```python
from build123d import *

# Parameters (mm, degrees)
SKETCH_W        = 55.5
SKETCH_H        = 55.5
SKETCH_R        = 19.25
PAD_DEPTH       = 6
SKETCH001_W     = 58.5
SKETCH001_H     = 8
PAD001_DEPTH    = 5
SKETCH002_W     = 30
SKETCH002_H     = 5
PAD002_DEPTH    = 20
FILLET_R        = 5
POCKET_DEPTH    = 6
FILLET001_R     = 9
FILLET002_R     = 7
CHAMFER_SIZE    = 3
SKETCH004_R     = 19.25
SKETCH004_R_2   = 18.5
PAD003_DEPTH    = 1.5
SKETCH005_W     = 45.5
SKETCH005_H     = 45.5
POCKET001_DEPTH = 3
SKETCH006_R     = 1
POCKET002_DEPTH = 6
FILLET003_R     = 1
FILLET004_R     = 1
SKETCH007_R     = 5
POCKET003_DEPTH = 2.999


with BuildPart() as part:
    # Sketch → Pad (new body)
    with BuildSketch(Plane.XY):
        Rectangle(SKETCH_W, SKETCH_H)
        Circle(SKETCH_R, mode=Mode.SUBTRACT)
    extrude(amount=PAD_DEPTH)

    # Sketch001 → Pad001 (new body)
    with BuildSketch(Plane(origin=(0, 27.75, 0), x_dir=(-1, 0, 0), z_dir=(0, 1, 0))):
        with Locations((0, 3)):
            Rectangle(SKETCH001_W, SKETCH001_H)
    extrude(amount=PAD001_DEPTH)

    # Sketch002 → Pad002 (new body)
    with BuildSketch(Plane(origin=(0, 32.75, 0), x_dir=(-1, 0, 0), z_dir=(0, 1, 0))):
        with Locations((0, 3)):
            Rectangle(SKETCH002_W, SKETCH002_H)
    extrude(amount=PAD002_DEPTH)

    # Fillet
    fillet_edges = [part.edges().sort_by_distance(p)[0] for p in [
        (-27.75, -27.75, 3),
        (27.75, -27.75, 3),
    ]]
    fillet(fillet_edges, radius=FILLET_R)

    # Sketch003 → Pocket (cut)
    with BuildSketch(Plane(origin=(0, 0, 0.5), x_dir=(1, 0, 0), z_dir=(0, 0, -1))):
        with BuildLine():
            ThreePointArc((-5, -36.75), (-11, -42.75), (-5, -48.75))
            Line((-5, -48.75), (5, -48.75))
            ThreePointArc((5, -48.75), (11, -42.75), (5, -36.75))
            Line((-5, -36.75), (5, -36.75))
        make_face()
    extrude(amount=-POCKET_DEPTH, mode=Mode.SUBTRACT)

    # Fillet001
    fillet001_edges = [part.edges().sort_by_distance(p)[0] for p in [
        (15, 52.75, 3),
        (-15, 52.75, 3),
    ]]
    fillet(fillet001_edges, radius=FILLET001_R)

    # Fillet002
    fillet002_edges = [part.edges().sort_by_distance(p)[0] for p in [
        (15, 32.75, 3),
        (-15, 32.75, 3),
    ]]
    fillet(fillet002_edges, radius=FILLET002_R)

    # Chamfer
    chamfer_edges = [part.edges().sort_by_distance(p)[0] for p in [
        (-29.25, 32.75, 3),
        (29.25, 32.75, 3),
    ]]
    chamfer(chamfer_edges, length=CHAMFER_SIZE)

    # Sketch004 → Pad003 (new body)
    with BuildSketch(Plane(origin=(0, 0, 0), x_dir=(1, 0, 0), z_dir=(0, 0, -1))):
        Circle(SKETCH004_R)
        Circle(SKETCH004_R_2, mode=Mode.SUBTRACT)
    extrude(amount=-PAD003_DEPTH)

    # Sketch005 → Pocket001 (cut)
    with BuildSketch(Plane.XY.offset(6)):
        Rectangle(SKETCH005_W, SKETCH005_H)
    extrude(amount=-POCKET001_DEPTH, mode=Mode.SUBTRACT)

    # Sketch006 → Pocket002 (cut)
    with BuildSketch(Plane.XY.offset(3)):
        with Locations((-18.40304, 10.625)):
            Circle(SKETCH006_R)
        with Locations((18.40304, 10.625)):
            Circle(SKETCH006_R)
        with Locations((0, -21.25)):
            Circle(SKETCH006_R)
    extrude(amount=-POCKET002_DEPTH, mode=Mode.SUBTRACT)

    # Fillet003
    fillet003_edges = [part.edges().sort_by_distance(p)[0] for p in [
        (0, 48.75, 5.5),
    ]]
    fillet(fillet003_edges, radius=FILLET003_R)

    # Fillet004
    fillet004_edges = [part.edges().sort_by_distance(p)[0] for p in [
        (0, 36.75, 0.5),
    ]]
    fillet(fillet004_edges, radius=FILLET004_R)

    # Sketch007 → Pocket003 (cut)
    with BuildSketch(Plane.XY.offset(6)):
        with Locations((0, -21.25)):
            Circle(SKETCH007_R)
    extrude(amount=-POCKET003_DEPTH, mode=Mode.SUBTRACT)


solid = part.part
```
Verification items for the finished model (mm, model axes). A direction names the side the tool comes from. Round coordinates to 2 decimals unless told otherwise and drop trailing zeros. Order: outer loops, then holes, each group sorted by start corner. A loop starts at its lowest first (then second) coordinate and runs counter-clockwise, first axis right, second up. Notation, with made-up numbers: (-8.75, -31.75) -> (-3.75, -31.75) arc R4 cw to (-3.75, -26.75) -> close; hole circle Ø1 at (-24.75, 26.25). An arc over 180 degrees is marked (long way). Put each result on its own line as item: value. Start each with the question number.
(1) Section check D-D (y = 14.5). Enter the section's corners in (x, z), then the cut area to 3 significant figures.
(2) Depth check by flat-ended pin: pin 1 Ø3 at (y, z) = (-1, 3) entering from +X; pin 2 Ø1.5 at (y, z) = (25, 1.5) entering from -X; pin 3 Ø10 at (x, y) = (-18, 5.5) entering from -Z. Enter the tip coordinate at first touch or a pass-through.
(3) Tool access check on faces 1 (the face through (0, 35, 5.5)), 2 (the face through (0, 36.75, 3)), 3 (the face through (-27.75, 2, 3)). Record the directions out of +Z, -Z, +X, -X, +Y, -Y that give a thin tool (end or side, any length) a straight path to the whole face; none if there is none.
(4) Material ranges on line 1 along Y through (x, z) = (0, 1.35); line 2 along Y through (x, z) = (0, 1.75); line 3 along X through (y, z) = (0, 1), recorded low to high.
(5) Draft check along X on faces 4 (the face through (-16, -10, 1.5)), 5 (the face through (-29.25, 29, 3)), 6 (the face through (0, 32.75, 0)). Enter one of: +X half, -X half, draft (parallel to the pull), parting line (faces both ways), or undercut.
(6) Section check B-B (x = 2). State how many separate pieces and enclosed holes the cut face has, then the cut area to 3 significant figures.
(7) Section check A-A (y = -21.25). Enter the section's corners in (x, z).
(8) Section check C-C (y = 42.75). Enter the section's corners in (x, z).
Completed:
1. outline: (-27.75, 0) -> (-11.49, 0) -> (-11.49, 1.5) -> (-12.66, 1.5) -> (-12.66, 3) -> (-22.75, 3) -> (-22.75, 6) -> (-27.75, 6) -> close; (11.49, 0) -> (27.75, 0) -> (27.75, 6) -> (22.75, 6) -> (22.75, 3) -> (12.66, 3) -> (12.66, 1.5) -> (11.49, 1.5) -> close
1. area: 124 mm2
2. pin 1: stops at x = 27.75
2. pin 2: stops at x = -27.75
2. pin 3: stops at z = 0
3. face 1: +Z, +X, -X, +Y
3. face 2: +Z, -Z
3. face 3: +Z, -Z, -X, -Y
4. line 1: y = -27.75 to -22.25, -20.25 to -18.5, 18.5 to 36.74, 48.76 to 52.75
4. line 2: y = -27.75 to -22.25, -20.25 to -19.25, 19.25 to 36.75, 48.75 to 52.75
4. line 3: x = -27.75 to -18.5, 18.5 to 27.75
5. face 4: undercut
5. face 5: -X half
5. face 6: draft
6. separate pieces: 3
6. enclosed holes: 0
6. area: 154 mm2
7. outline: (-27.75, 0) -> (-1, 0) -> (-1, 3) -> (-22.75, 3) -> (-22.75, 6) -> (-27.75, 6) -> close; (1, 0) -> (27.75, 0) -> (27.75, 6) -> (22.75, 6) -> (22.75, 3) -> (1, 3) -> close
8. outline: (-15, 0.5) -> (-12, 0.5) arc R1 ccw to (-11, 1.5) -> (-11, 4.5) arc R1 ccw to (-12, 5.5) -> (-15, 5.5) -> close; (11, 1.5) arc R1 ccw to (12, 0.5) -> (15, 0.5) -> (15, 5.5) -> (12, 5.5) arc R1 ccw to (11, 4.5) -> close
